from build123d import *

# Parameters (mm, degrees)
SKETCH_R     = 1.25
SKETCH_R_2   = 12
PAD_DEPTH    = 3
SKETCH001_W  = 42.3
SKETCH001_H  = 3
PAD001_DEPTH = 48
SKETCH002_R  = 3
SKETCH002_W  = 15
SKETCH002_H  = 15
POCKET_DEPTH = 48.301


with BuildPart() as part:
    # Sketch → Pad (new body)
    with BuildSketch(Plane.XY):
        Polygon((0, 0), (42.3, 0), (42.3, 42.3), (42.3, 48.3), (0, 48.3), (0, 42.3), align=None)
        with Locations((5.65, 36.65)):
            Circle(SKETCH_R, mode=Mode.SUBTRACT)
        with Locations((36.65, 36.65)):
            Circle(SKETCH_R, mode=Mode.SUBTRACT)
        with Locations((5.65, 5.65)):
            Circle(SKETCH_R, mode=Mode.SUBTRACT)
        with Locations((36.65, 5.65)):
            Circle(SKETCH_R, mode=Mode.SUBTRACT)
        with Locations((21.15, 21.15)):
            Circle(SKETCH_R_2, mode=Mode.SUBTRACT)
    extrude(amount=PAD_DEPTH)

    # Sketch001 → Pad001 (new body)
    with BuildSketch(Plane(origin=(0, 0, 0), x_dir=(1, 0, 0), z_dir=(0, 0, -1))):
        with Locations((21.15, -46.8)):
            Rectangle(SKETCH001_W, SKETCH001_H)
    extrude(amount=PAD001_DEPTH)

    # Sketch002 → Pocket (cut, through all)
    with BuildSketch(Plane(origin=(0, 48.3, 0), x_dir=(-1, 0, 0), z_dir=(0, 1, 0))):
        with Locations((-36.3, -7)):
            Circle(SKETCH002_R)
        with Locations((-6, -7)):
            Circle(SKETCH002_R)
        with Locations((-36.3, -38)):
            Circle(SKETCH002_R)
        with Locations((-6, -38)):
            Circle(SKETCH002_R)
        with Locations((-21.15, -40.5)):
            Rectangle(SKETCH002_W, SKETCH002_H)
    extrude(amount=-POCKET_DEPTH, mode=Mode.SUBTRACT)


solid = part.part
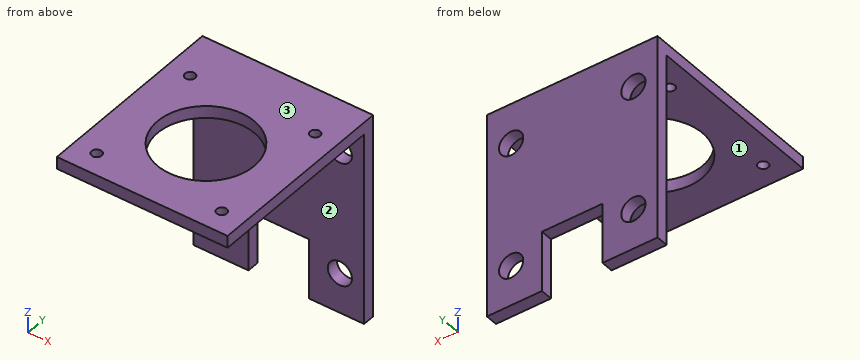
Model file for the job. Use its own axes, mm. Face numbers are marked on the shaded views. Give positions to 0.01 mm unless a question says otherwise; leave off trailing zeros. Order: outer loops, then holes, each group sorted by start corner. A loop starts at its lowest first (then second) coordinate and runs counter-clockwise, first axis right, second up. Notation, with made-up numbers: M 15,-35.5 L 26,-35.5 A19 ccw 26,-17.5 Z; hole C 62.5,68.5 d6. An arc over 180 degrees is marked long. Put each result on its own line as item: value. Start each with the question number.
(1) Drill centre lines: L1, parallel to Z at x = 6, y = 47.7; L2, parallel to Y at x = 21.15, z = 0.9; L3, parallel to Y at x = 36.65, z = 2. Where is each one in solid material? Low to high. Write a range as [from, to].
(2) Band-saw the part on C-C on z = -36. Give the cut face in (x, y).
(3) Pin check, flat tips, straight feed: pin 1 Ø9.5 at (x, z) = (6, -38) entering from +Y; pin 2 Ø2 at (x, y) = (20, 7.5) entering from -Z; pin 3 Ø8 at (x, z) = (6, -7) entering from -Y; pin 4 Ø1.5 at (x, y) = (5.65, 5.65) entering from -Z. Stop position of each tip, or through.
(4) Pull direction Z, two halves, no side cores. Call the marked faces 1, 2 and 3: released by +Z, released by -Z, zero draft, split by the parting line, or undercut.
(5) Band-saw the part on B-B on y = 36.65. Give the cut face in (x, z), then the cut area to 3 significant figures.
(6) Band-saw the part on A-A on x = 21.15. Give the cut face in (y, z).
(7) Band-saw the part on D-D on y = 30. Give the cut face in (x, z), then the cut area to 3 significant figures.
Results below:
1. L1: z = [-48, -41], [-35, -10], [-4, 3]
1. L2: y = [0, 9.15], [33.15, 48.3]
1. L3: y = [0, 4.4], [6.9, 35.4], [37.9, 48.3]
2. outline: M 0,45.3 L 3.76,45.3 L 3.76,48.3 L 0,48.3 Z; M 8.24,45.3 L 13.65,45.3 L 13.65,48.3 L 8.24,48.3 Z; M 28.65,45.3 L 34.06,45.3 L 34.06,48.3 L 28.65,48.3 Z; M 38.54,45.3 L 42.3,45.3 L 42.3,48.3 L 38.54,48.3 Z
3. pin 1: stops at y = 48.3
3. pin 2: stops at z = 0
3. pin 3: stops at y = 45.3
3. pin 4: passes through
4. face 1: released by -Z
4. face 2: zero draft
4. face 3: released by +Z
5. outline: M 0,0 L 4.4,0 L 4.4,3 L 0,3 Z; M 6.9,0 L 35.4,0 L 35.4,3 L 6.9,3 Z; M 37.9,0 L 42.3,0 L 42.3,3 L 37.9,3 Z
5. area: 112 mm2
6. outline: M 0,0 L 9.15,0 L 9.15,3 L 0,3 Z; M 33.15,0 L 45.3,0 L 45.3,-33 L 48.3,-33 L 48.3,3 L 33.15,3 Z
7. outline: M 0,0 L 13.05,0 L 13.05,3 L 0,3 Z; M 29.25,0 L 42.3,0 L 42.3,3 L 29.25,3 Z
7. area: 78.3 mm2
